```python
from build123d import *

# Parameters (mm, degrees)
PAD_DEPTH    = 5
SKETCH001_R  = 1.5
POCKET_DEPTH = 4
SKETCH004_R  = 1.5
PAD001_DEPTH = 5


with BuildPart() as part:
    # Sketch → Pad (new body, symmetric)
    with BuildSketch(Plane.XY):
        Polygon((2.6, 1.501111), (0, 3.002221), (-2.6, 1.501111), (-2.6, -1.501111), (0, -3.002221), (2.6, -1.501111), align=None)
    extrude(amount=PAD_DEPTH, both=True)

    # Sketch001 (on Face8 of Pad) → Pocket (cut)
    with BuildSketch(Plane.XY.offset(5)):
        Circle(SKETCH001_R)
    extrude(amount=-POCKET_DEPTH, mode=Mode.SUBTRACT)

    # Sketch004 (on Face4 of Pocket) → Pad001 (join)
    with BuildSketch(Plane(origin=(0, 0, -5), x_dir=(1, 0, 0), z_dir=(0, 0, -1))):
        Circle(SKETCH004_R)
    extrude(amount=PAD001_DEPTH)

    # Sketch005 → Groove (revolve, cut)
    with BuildSketch(Plane.YZ):
        Polygon((1.8, 5.75), (5.8, 5.75), (5.8, -5.75), (1.8, -5.75), (4.05, -3.5), (4.05, 3.5), align=None)
    revolve(axis=Axis((0, 0, 0), (0, 0, 1)), mode=Mode.SUBTRACT)


solid = part.part
```
The listing builds one solid part. Answer for the finished solid, in the listing's coordinates (mm). A direction names the side the tool comes from. Round coordinates to 2 decimals unless told otherwise and drop trailing zeros. Loops run counter-clockwise (first coordinate to the right, second up) from the corner with the lowest first, then second, coordinate; pieces in that order, holes last.
1) A cutting plane is placed at B-B on y = 0. Determine the outline of the cut face in (x, z), plus the area to 3 significant figures.
Outcome:
outline: (-2.6, -4.95) - (-2.55, -5) - (-1.5, -5) - (-1.5, -10) - (1.5, -10) - (1.5, -5) - (2.55, -5) - (2.6, -4.95) - (2.6, 4.95) - (2.55, 5) - (1.5, 5) - (1.5, 1) - (-1.5, 1) - (-1.5, 5) - (-2.55, 5) - (-2.6, 4.95) - close
area: 55.0 mm2
2) A cutting plane is placed at C-C on z = -1.75. Determine the outline of the cut face in (x, y).
Outcome:
outline: (-2.6, -1.5) - (0, -3) - (2.6, -1.5) - (2.6, 1.5) - (0, 3) - (-2.6, 1.5) - close
3) For a pull along Y with two mould halves and no side action, classify faces 1 (the face through (-1.32, -2.24, 0.07)), 2 (the face through (-2.6, 0, 0)), 3 (the face through (-1.5, 0.07, 3.03)) as released by +Y, released by -Y, zero draft, split by the parting line, or undercut.
Outcome:
face 1: released by -Y
face 2: zero draft
face 3: undercut
4) Consider line 1 (Z direction, x = -0.35, y = 1.5); line 2 (Z direction, x = 0.15, y = 1); line 3 (Y direction, x = -0.6, z = -3.5). Determine where each line is inside the solid, lowest interval first.
Outcome:
line 1: z = -5 to 5
line 2: z = -10 to 1
line 3: y = -2.66 to 2.66
5) A cutting plane is placed at A-A on z = 1.5. Determine the outline of the cut face in (x, y), plus the area to 3 significant figures.
Outcome:
outline: (-2.6, -1.5) - (0, -3) - (2.6, -1.5) - (2.6, 1.5) - (0, 3) - (-2.6, 1.5) - close; hole circle Ø3 at (0, 0)
area: 16.3 mm2
6) Given P1, Ø2.5, axis at x = 0, y = 0, coming from the +Z side, flat-ended and moving along its own axis, determine where the tip first touches the part or whether it passes through.
Outcome:
P1: stops at z = 1
7) A cutting plane is placed at D-D on z = -7. Determine the outline of the cut face in (x, y), plus the area to 3 significant figures.
Outcome:
outline: circle Ø3 at (0, 0)
area: 7.07 mm2
8) For faces 4 (the face through (0, -2, -5)), 5 (the face through (1.32, 2.24, 0.07)), 6 (the face through (0, 0, 1)), determine the directions among +Z, -Z, +X, -X, +Y, -Y from which every point of the face is accessible in a straight line to the end or side of a thin tool.
Outcome:
face 4: -Z
face 5: +Z, -Z, +X, +Y
face 6: +Z
